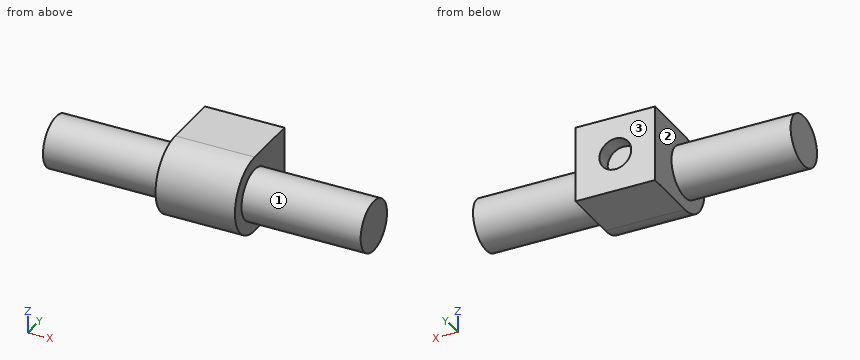
from build123d import *

# Parameters (mm, degrees)
BOSS_EXTRUDE1_DEPTH = 12.5
SKETCH2_R           = 8
BOSS_EXTRUDE2_DEPTH = 50
SKETCH3_R           = 5
CUT_EXTRUDE1_DEPTH  = 5


with BuildPart() as part:
    # Sketch1 → Boss-Extrude1 (new body, symmetric)
    with BuildSketch(Plane(origin=(0, 0, 0), x_dir=(0, 0, -1), z_dir=(1, 0, 0))):
        with BuildLine():
            Line((-12, 0), (-12, 18))
            Line((-12, 18), (12, 18))
            Line((12, 18), (12, 0))
            ThreePointArc((12, 0), (0, -12), (-12, 0))
        make_face()
    extrude(amount=BOSS_EXTRUDE1_DEPTH, both=True)

    # Sketch2 → Boss-Extrude2 (add, symmetric)
    with BuildSketch(Plane(origin=(0, 0, 0), x_dir=(0, 0, -1), z_dir=(1, 0, 0))):
        Circle(SKETCH2_R)
    extrude(amount=BOSS_EXTRUDE2_DEPTH, both=True)

    # Sketch3 → Cut-Extrude1 (cut)
    with BuildSketch(Plane(origin=(0, 18, 0), x_dir=(1, 0, 0), z_dir=(0, 1, 0))):
        Circle(SKETCH3_R)
    extrude(amount=-CUT_EXTRUDE1_DEPTH, mode=Mode.SUBTRACT)


solid = part.part
Can you work these out from the model? Positions are in its coordinate system, mm. Face numbers are marked on the shaded views. A direction names the side the tool comes from. Coordinates: 2 decimals unless noted, no trailing zeros. Loops run counter-clockwise (first coordinate to the right, second up) from the corner with the lowest first, then second, coordinate; pieces in that order, holes last. Notation, with made-up numbers: (-25.5, -12) - (-11.5, -12) arc R29 cw to (-11.5, 19) - close; hole circle Ø4 at (10.25, 86.5). An arc over 180 degrees is marked (long way). Answer as a JSON object with one key per item and string values. Group by question number.
Item 1: If I drill on L1, parallel to X at y = 15.8, z = 0; L2, parallel to Z at x = 0, y = 16; L3, parallel to Y at x = -28, z = 6.25, over which ranges is the centre line in solid material (lowest first)? Write a range as from..to.
Item 2: On a 3-axis mill with a long thin cutter (end or side, diameter ignored), from which of +Z, -Z, +X, -X, +Y, -Y can I reach the whole of each face in a straight line? I mean the marked faces 1, 2 and 3. Say none if no direction works.
Item 3: If we section it at D-D (y = 2): List the corners of the cut face in (x, z) for me, plus the area to 3 significant figures.
Item 4: If we section it at B-B (y = 14.5): List the corners of the cut face in (x, z) for me.
Item 5: For pin 1 (10 mm diameter, centred on x = -22, y = 6.5, fed in from -Z); pin 2 (5 mm diameter, centred on y = 11, z = 7, fed in from +X); pin 3 (5 mm diameter, centred on x = 17.5, y = -8.5, fed in from +Z), each with a flat end and sliding along its axis, tell me the tip position at first contact or that it passes through.
Item 6: If we section it at C-C (z = 0): List the corners of the cut face in (x, y) for me.
Item 7: If we section it at A-A (x = 0): List the corners of the cut face in (y, z) for me, plus the area to 3 significant figures.
Returned:
{
 "1": {"L1": "x = -12.5..-5, 5..12.5", "L2": "z = -12..-5, 5..12", "L3": "y = -4.99..4.99"},
 "2": {"face 1": "+X", "face 2": "-X", "face 3": "+Z, -Z, +X, -X, +Y"},
 "3": {"outline": "(-50, -7.75) - (-12.5, -7.75) - (-12.5, -12) - (12.5, -12) - (12.5, -7.75) - (50, -7.75) - (50, 7.75) - (12.5, 7.75) - (12.5, 12) - (-12.5, 12) - (-12.5, 7.75) - (-50, 7.75) - close", "area": "1,760 mm²"},
 "4": {"outline": "(-12.5, -12) - (12.5, -12) - (12.5, 12) - (-12.5, 12) - close; hole circle Ø10 at (0, 0)"},
 "5": {"pin 1": "stops at z = -7.86", "pin 2": "stops at x = 12.5", "pin 3": "stops at z = 5.29"},
 "6": {"outline": "(-50, -8) - (-12.5, -8) - (-12.5, -12) - (12.5, -12) - (12.5, -8) - (50, -8) - (50, 8) - (12.5, 8) - (12.5, 18) - (5, 18) - (5, 13) - (-5, 13) - (-5, 18) - (-12.5, 18) - (-12.5, 8) - (-50, 8) - close"},
 "7": {"outline": "(0, -12) - (18, -12) - (18, -5) - (13, -5) - (13, 5) - (18, 5) - (18, 12) - (0, 12) arc R12 ccw to start", "area": "608 mm²"}
}
